Design review of the part shown in the three views and the two pictorial views. Dimensions are in mm from the part's minimum x, y and z. Give positions to 0.01 mm unless a question says otherwise; leave off trailing zeros. Write each loop counter-clockwise with the first axis right and the second up, starting at its lowest first coordinate (ties: lowest second). Pieces come first, ordered by that corner, then holes. Notation, with made-up numbers: M 57.25,-29.5 L 95.25,-29.5 A20 cw 95.25,3.5 Z; hole C 63,17 d10. An arc over 180 degrees is marked long. Write item = value, one per line.
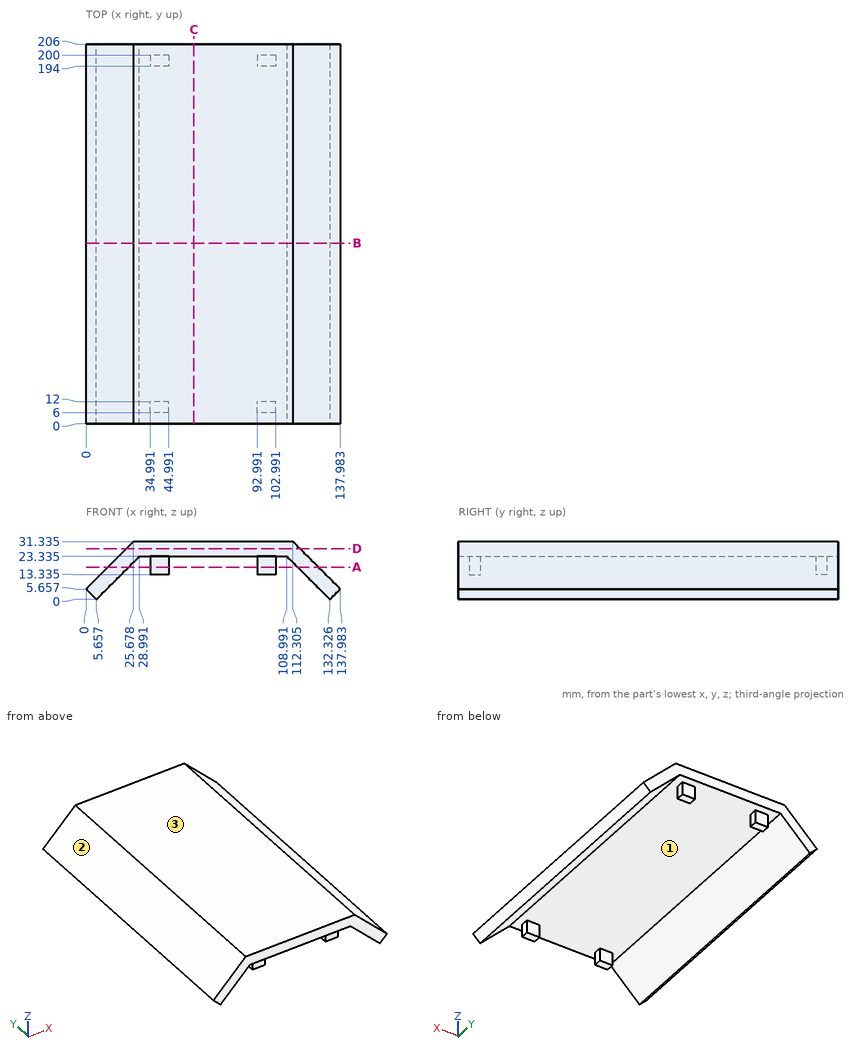
1. We need section D-D, the plane z = 27.5. Write out the cut boundary in (x, y), then the cut area to 3 significant figures.
Responses:
outline = M 21.84,0 L 116.14,0 L 116.14,206 L 21.84,206 Z
area = 19,400 mm2
2. We need section B-B, the plane y = 98. Write out the cut boundary in (x, z) (1 decimal).
Responses:
outline = M 0,5.7 L 5.7,0 L 29,23.3 L 109,23.3 L 132.3,0 L 138,5.7 L 112.3,31.3 L 25.7,31.3 Z
3. We need section A-A, the plane z = 17.5. Write out the cut boundary in (x, y) (1 decimal), then the cut area to 3 significant figures.
Responses:
outline = M 11.8,0 L 23.2,0 L 23.2,206 L 11.8,206 Z; M 35,6 L 45,6 L 45,12 L 35,12 Z; M 35,194 L 45,194 L 45,200 L 35,200 Z; M 93,6 L 103,6 L 103,12 L 93,12 Z; M 93,194 L 103,194 L 103,200 L 93,200 Z; M 114.8,0 L 126.1,0 L 126.1,206 L 114.8,206 Z
area = 4,900 mm2
4. The part is to be moulded in two halves that separate along X. For the marked faces 1, 2 and 3, say which applies: +X half, -X half, draft (parallel to the pull), parting line (faces both ways), or undercut.
Responses:
face_1 = undercut
face_2 = -X half
face_3 = draft
5. We need section C-C, the plane x = 58.5. Write out the cut boundary in (y, z) (1 decimal), then the cut area to 3 significant figures.
Responses:
outline = M 0,23.3 L 206,23.3 L 206,31.3 L 0,31.3 Z
area = 1,650 mm2
6. Insertion check: P1, Ø3, axis at x = 96.5, z = 16, coming from the -Y side; P2, Ø6, axis at y = 165.5, z = 4, coming from the +X side; P3, Ø6.5, axis at x = 39, y = 10, coming from the -Z side (1 decimal); P4, Ø6.5, axis at y = 10.5, z = 18.5, coming from the -X side (1 decimal). Each pin has a flat end and moves straight along its axis. Give the tip position at first contact, or say it passes through.
Responses:
P1 = 6
P2 = 137.98
P3 = 13.3
P4 = 9.6
7. For line 1 along X through (y, z) = (197.5, 19) (1 decimal); line 2 along Z through (x, y) = (47, 35) (1 decimal); line 3 along Y through (x, z) = (38, 23), list the stretches that pass through material, from the lowest coordinate up. Write a range as from..to.
Responses:
line_1 = 13.3..24.7, 35..45, 93..103, 113.3..124.6
line_2 = 23.3..31.3
line_3 = 6..12, 194..200
